Autodesk Inventor part; units mm, degrees
ref_plane "YZ Plane" through (0, 0, 0) normal (1, 0, 0) x (0, 1, 0)
ref_plane "XZ Plane" through (0, 0, 0) normal (0, 1, 0) x (-1, 0, 0)
ref_plane "XY Plane" through (0, 0, 0) normal (0, 0, 1) x (1, 0, 0)
sketch "Sketch1" plane through (0, 0, 0) normal (0, 0, 1) x (1, 0, 0)
  line L0 (15, -7.5) -> (-15, -7.5)
  line L1 (-15, -7.5) -> (-15, 7.5)
  line L2 (-15, 7.5) -> (15, 7.5)
  line L3 (15, 7.5) -> (15, -7.5)
  line L4 (15, -7.5) -> (-15, 7.5) construction
  line L5 (-15, -7.5) -> (15, 7.5) construction
  point P0 (0, 0)
  dimension "d0" = 15
  dimension "d1" = 30
extrude "Extrusion1" add sketch "Sketch1" along normal blind 18
sketch "Sketch2" plane through (-15, 7.5, 0) normal (0, 1, 0) x (1, 0, 0)
  line L0 (30, 0) -> (0, 0)
  line L1 (0, 0) -> (0, -18)
  line L2 (30, -18) -> (0, -18)
  line L3 (30, 0) -> (30, -18)
  circle A0 centre (7.5, -12) radius 5.25
  circle A1 centre (22.5, -12) radius 5.25
  line L4 (30, 0) -> (0, 0)
  point P0 (15, 0)
  point P1 (15, 0)
  point P2 (15, 0)
  dimension "d4" = 10.5
  dimension "d5" = 6
  dimension "d6" = 7.5
  dimension "d7" = 7.5
extrude "Extrusion2" cut sketch "Sketch2" against normal blind 2 contours A0 | A1
chamfer "Chamfer1" distance 3 angle 45 2 edges at (15, 0, 18) (-15, 0, 18)
sketch "Sketch3" plane through (0, 0, 18) normal (0, 0, 1) x (1, 0, 0)
  line L0 (-12, -7.5) -> (-12, 7.5)
  line L1 (-12, -7.5) -> (12, -7.5)
  line L2 (12, 7.5) -> (12, -7.5)
  line L3 (12, 7.5) -> (-12, 7.5)
  point P0 (0, 0)
  point P1 (-7.5, 0)
  point P2 (7.5, 0)
  dimension "d13" = 7.5
  dimension "d14" = 7.5
hole "Hole1" at (-7.5, 0, 18) at (7.5, 0, 18) direction (0, 0, -1) diameter 3.6 end through all counterbore diameter 6.5 counterbore depth 9
properties part number "Door Base Magnet" material "ABS Plastic"
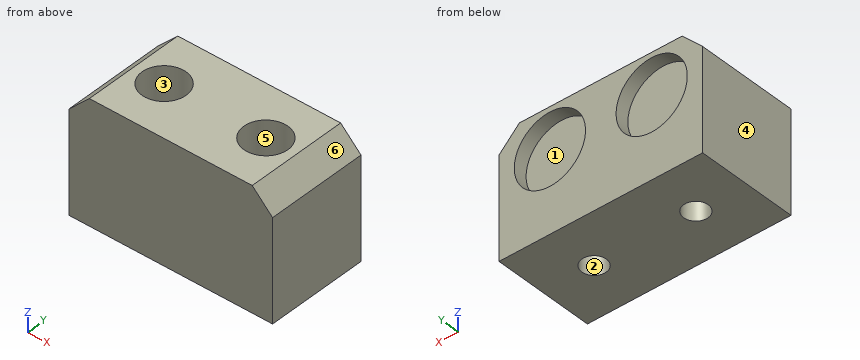
Check sheet for the modelled part. Datum: model origin and axes. Units: mm. Face numbers are marked on the shaded views. A direction names the side the tool comes from. Round coordinates to 2 decimals unless told otherwise and drop trailing zeros. Loops run counter-clockwise (first coordinate to the right, second up) from the corner with the lowest first, then second, coordinate; pieces in that order, holes last. Notation, with made-up numbers: M -28.75,57.25 L 25.25,57.25 A24 cw 25.25,78.25 Z; hole C -14.75,52 d3. An arc over 180 degrees is marked long. One line per item, written item: value.
(1) Thickness scan on line 1 (X direction, y = 6.7, z = 12); line 2 (X direction, y = 0, z = 14); line 3 (Y direction, x = -7.5, z = 7). Record the ranges inside material, lowest first.
Computed values:
line 1: x = -15 to -12.75, -2.25 to 2.25, 12.75 to 15
line 2: x = -15 to -10.75, -4.25 to 4.25, 10.75 to 15
line 3: y = -7.5 to -1.8, 1.8 to 5.5
(2) Sectioned sample at B-B, the plane z = 12. Record the cut outline in (x, y), then the cut area to 3 significant figures.
Computed values:
outline: M -15,-7.5 L 15,-7.5 L 15,7.5 L 12.75,7.5 L 12.75,5.5 L 2.25,5.5 L 2.25,7.5 L -2.25,7.5 L -2.25,5.5 L -12.75,5.5 L -12.75,7.5 L -15,7.5 Z; hole C -7.5,0 d6.5; hole C 7.5,0 d6.5
area: 342 mm^2
(3) Access from +Z, -Z, +X, -X, +Y, -Y to the whole of each face (thin tool, end or side, straight path). Record for the marked faces 1, 2 and 3.
Computed values:
face 1: +Y
face 2: +Z, -Z
face 3: +Z
(4) Depth check by flat-ended pin: pin 1 Ø2 at (x, y) = (-7, -1.5) entering from +Z; pin 2 Ø2 at (x, y) = (7.5, 0) entering from +Z (3 decimals); pin 3 Ø9.5 at (x, z) = (7.5, 12) entering from +Y. Enter the tip coordinate at first touch or a pass-through.
Computed values:
pin 1: stops at z = 9
pin 2: passes through
pin 3: stops at y = 5.5
(5) Release check for a two-part mould opening along X. For the marked faces 4, 5 and 6 record: +X half, -X half, draft (parallel to the pull), parting line (faces both ways), or undercut.
Computed values:
face 4: -X half
face 5: undercut
face 6: +X half
(6) Sectioned sample at D-D, the plane y = 2.25. Record the cut outline in (x, z).
Computed values:
outline: M -15,0 L 15,0 L 15,15 L 12,18 L 9.85,18 L 9.85,9 L 5.15,9 L 5.15,18 L -5.15,18 L -5.15,9 L -9.85,9 L -9.85,18 L -12,18 L -15,15 Z
(7) Sectioned sample at A-A, the plane x = 7.5. Record the cut outline in (y, z).
Computed values:
outline: M -7.5,0 L -1.8,0 L -1.8,9 L -3.25,9 L -3.25,18 L -7.5,18 Z; M 1.8,0 L 7.5,0 L 7.5,6.75 L 5.5,6.75 L 5.5,17.25 L 7.5,17.25 L 7.5,18 L 3.25,18 L 3.25,9 L 1.8,9 Z
(8) Sectioned sample at C-C, the plane y = 0. Record the cut outline in (x, z).
Computed values:
outline: M -15,0 L -9.3,0 L -9.3,9 L -10.75,9 L -10.75,18 L -12,18 L -15,15 Z; M -5.7,0 L 5.7,0 L 5.7,9 L 4.25,9 L 4.25,18 L -4.25,18 L -4.25,9 L -5.7,9 Z; M 9.3,0 L 15,0 L 15,15 L 12,18 L 10.75,18 L 10.75,9 L 9.3,9 Z
